The listing builds one solid part. Answer for the finished solid, in the listing's coordinates (mm). Coordinates: 2 decimals unless noted, no trailing zeros. Write each loop counter-clockwise with the first axis right and the second up, starting at its lowest first coordinate (ties: lowest second). Pieces come first, ordered by that corner, then holes.
Autodesk Inventor part; units mm, degrees
ref_plane "Work Plane1" through (-12.0937, 0, 0) normal (0, -0.8660254, -0.5) x (1, 0, 0)
ref_plane "YZ Plane" through (0, 0, 0) normal (1, 0, 0) x (0, 1, 0)
ref_plane "XZ Plane" through (0, 0, 0) normal (0, 1, 0) x (-1, 0, 0)
sketch "Sketch1" plane through (0, 0, 0) normal (1, 0, 0) x (0, 1, 0)
  line L0 (-5.7735, 0) -> (-2.8868, 5)
  line L1 (-2.8868, 5) -> (2.8868, 5)
  line L2 (2.8868, 5) -> (5.7735, 0)
  line L3 (5.7735, 0) -> (2.8868, -5)
  line L4 (2.8868, -5) -> (-2.8868, -5)
  line L5 (-2.8868, -5) -> (-5.7735, 0)
  point P0 (0, 0)
  point P1 (0, 0)
  dimension "d0" = 11.547
extrude "Body" add sketch "Sketch1" along normal blind 3.6
sketch "Sketch2" plane through (0, 0, 0) normal (0, 0, 1) x (1, 0, 0)
  line L0 (0, 2.8868) -> (0, 5.7735)
  line L1 (0, 5.7735) -> (3.6, 5.7735)
  line L2 (3.6, 2.8868) -> (3.6, 5.7735)
  line L3 (-0.72, 0) -> (4.32, 0)
  line L4 (0.4466, 5.7735) -> (0, 5)
  line L5 (3.1534, 5.7735) -> (3.6, 5)
  dimension "d3" = 30
  dimension "d4" = 30
  dimension "d5" = 10
  dimension "d6" = 10
revolve "Chamfer1" cut sketch "Sketch2" angle 360 about axis through (-10, 0, 0) along (1, 0, 0)
sketch "Sketch3" plane through (3.6, 0, 0) normal (1, 0, 0) x (0, 0, -1)
  arc A0 (-2.5, -4.3301) -> (2.5, -4.3301) centre (0, 0) ccw
hole "Thread" at (3.6, 0, 0) direction (-1, 0, 0) diameter 4.917 end through all
chamfer "Chamfer2" distance 0.5413 angle 30 1 edges at (3.6, 0, 2.4585) measured on face at (3.6, 4.1286, -0.0988)
chamfer "Chamfer3" distance 0.5413 angle 30 1 edges at (0, 0, 2.4585) measured on face at (0, 4.1286, -0.0988)
ref_plane "Work Plane1" through (-12.0937, 0, 0) normal (0, -0.8660254, -0.5) x (1, 0, 0)
equation "\"d0\" = 1.1547 * SW"
equation "\"d1\" = KOH"
equation "\"d8\" = -0.5 * GD1 + 0.5 * NND"
equation "\"d40\" = -0.5 * GD1 + 0.5 * NND"
equation "\"d10\" = -0.5 * GD1 + 0.5 * NND"
equation "\"d41\" = -0.5 * GD1 + 0.5 * NND"
equation "\"d3\" = ANG1"
equation "\"d4\" = ANG2"
equation "\"d5\" = SW0"
equation "\"d6\" = SW01"
equation "\"ANG1\" = 30deg"
equation "\"ANG2\" = 30deg"
equation "\"NND\" = 6"
equation "\"KOH\" = 3.6"
equation "\"SW0\" = SW"
equation "\"SW01\" = SW"
equation "\"GUL\" = 0.541266 * PTC"
equation "\"THREADDIA\" = 6"
equation "\"TOA\" = 30deg"
equation "\"PTC\" = 1"
equation "\"E0\" = 1.155 * SW"
equation "\"GAL\" = 0.541266 * PTC"
properties part number "AS 1112 - M6" material "Steel, Mild"
(1) For a pull along Z with two mould halves and no side action, classify faces 1 (the cylindrical face through (1.779, -0.738, -2.345)), 2 (the conical face through (0.11, 5.19, -0.01)), 3 (the flat face through (1.775, -4.35, 2.465)) as pulls with the +Z half, pulls with the -Z half, needs draft (parallel to the pull), parting line crosses it, or undercut.
(2) Find the intervals of material crossed by probe 1 along Z at (x, y) = (1.7, 0); probe 2 along Y at (x, z) = (0.55, -0.5); probe 3 along Y at (x, z) = (0.25, -0.25), in increasing order.
(3) Each of these flat-tipped pins is pushed along its axis until it touches: pin 1 (1.5 mm diameter, centred on x = 3, z = -2, fed in from +Y); pin 2 (5.5 mm diameter, centred on y = 0, z = 0, fed in from -X); pin 3 (1 mm diameter, centred on x = 3, y = -4, fed in from +Z). Where does it stop, or does it pass through?
(4) Section A-A, the plane x = 2.55 is taken. Write down the section's boundary in (y, z), plus the area to 3 significant figures.
Solution:
1. face 1: undercut
1. face 2: parting line crosses it
1. face 3: pulls with the +Z half
2. probe 1: z = -5 to -2.46, 2.46 to 5
2. probe 2: y = -5.48 to -2.41, 2.41 to 5.48
2. probe 3: y = -5.43 to -2.55, 2.55 to 5.43
3. pin 1: stops at y = 5.05
3. pin 2: stops at x = 0.14
3. pin 3: stops at z = 3.94
4. outline: (-5.77, 0) - (-2.89, -5) - (2.89, -5) - (5.77, 0) - (2.89, 5) - (-2.89, 5) - close; hole circle Ø4.92 at (0, 0)
4. area: 67.6 mm2
